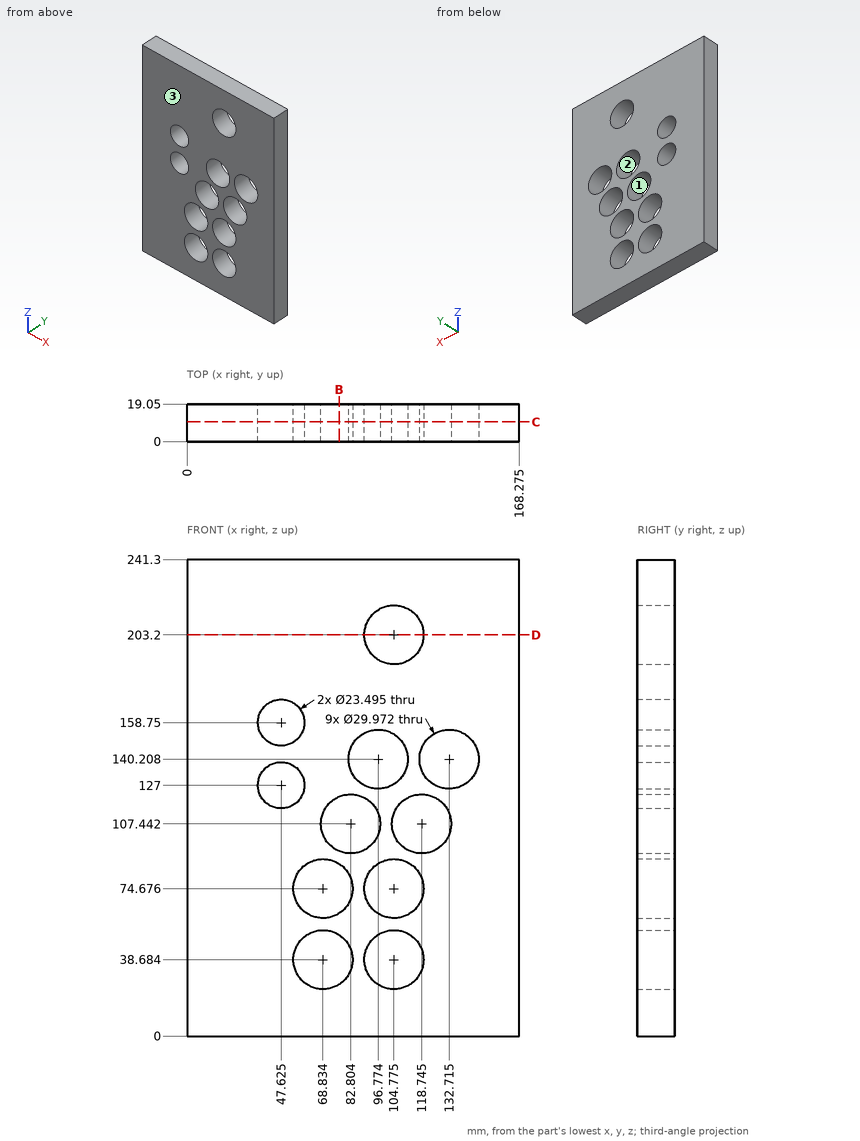
Answer from the drawing. Dimensions are ordinates in mm from the lowest x, y and z of the part. Coordinates: 2 decimals unless noted, no trailing zeros. Loops run counter-clockwise (first coordinate to the right, second up) from the corner with the lowest first, then second, coordinate; pieces in that order, holes last.
1) Section B-B (x = 77) is taken. Give the vertices of the cut face in (y, z), plus the area to 3 significant figures.
Results:
outline: (0, 0) - (19.05, 0) - (19.05, 26.12) - (0, 26.12) - close; (0, 51.25) - (19.05, 51.25) - (19.05, 62.11) - (0, 62.11) - close; (0, 87.24) - (19.05, 87.24) - (19.05, 93.63) - (0, 93.63) - close; (0, 121.26) - (19.05, 121.26) - (19.05, 241.3) - (0, 241.3) - close
area: 3,110 mm2
2) For a pull along Z with two mould halves and no side action, classify the marked faces 1, 2 and 3 as +Z half, -Z half, draft (parallel to the pull), parting line (faces both ways), or undercut.
Results:
face 1: undercut
face 2: undercut
face 3: draft
3) Consider probe 1 along Z at (x, y) = (46.5, 7.5); probe 2 along Z at (x, y) = (49.5, 16.5); probe 3 along Z at (x, y) = (57, 16.5). Determine where each line is inside the solid, lowest interval first.
Results:
probe 1: z = 0 to 115.31, 138.69 to 147.06, 170.44 to 241.3
probe 2: z = 0 to 115.4, 138.6 to 147.15, 170.35 to 241.3
probe 3: z = 0 to 29.49, 47.88 to 65.48, 83.87 to 119.92, 134.08 to 151.67, 165.83 to 241.3
4) Section C-C (y = 10) is taken. Give the number of separate pieces and of enclosed holes in the cut face, plus the area to 3 significant figures.
Results:
separate pieces: 1
enclosed holes: 11
area: 33,400 mm2
5) Section D-D (z = 203.2) is taken. Give the vertices of the cut face in (x, y) (3 decimals).
Results:
outline: (0, 0) - (89.789, 0) - (89.789, 19.05) - (0, 19.05) - close; (119.761, 0) - (168.275, 0) - (168.275, 19.05) - (119.761, 19.05) - close
